Could you check a few things on this drawing? It's one solid part, dimensions in mm from its lowest x, y, z. A direction names the side the tool comes from. Give positions to 0.01 mm unless a question says otherwise; leave off trailing zeros. Order: outer loops, then holes, each group sorted by start corner. A loop starts at its lowest first (then second) coordinate and runs counter-clockwise, first axis right, second up. Notation, with made-up numbers: (77, -24) -> (131, -24) arc R10 cw to (131, -20) -> close; hole circle Ø7 at (-23.75, -9). An arc over 180 degrees is marked (long way). Write each question's results on one line, items separated by ' | '. Start each with the question number.
Q1. Imagine slicing it at C-C, the plane x = 65.5. Please give me the cut outline in (y, z).
Q2. Imagine slicing it at B-B, the plane y = 338.5. Please give me the cut outline in (x, z).
Q3. Thinking about a two-plate mould opening in Z: for the marked faces 1, 2, 3 and 4, which applies, pulls with the +Z half, pulls with the -Z half, needs draft (parallel to the pull), parting line crosses it, or undercut?
Q4. I need wall thicknesses on line 1 along Z through (x, y) = (708, 216.5); line 2 along X through (y, z) = (122, 313). Which ranges of each line are inside material? Lowest first, please. Write a range as [from, to].
Q5. I'm going to push a flat-ended pin straight in: pin 1 (3 mm diameter, centred on y = 198.5, z = 313, fed in from -X). Where does the tip first touch, or does it pass through?
Q6. For the marked faces 5 and 6, which set-ups out of +Z, -Z, +X, -X, +Y, -Y let a thin tool reach every point of the face, with its end or its side?
Q7. Imagine slicing it at A-A, the plane z = 424. Please give me the cut outline in (x, y).
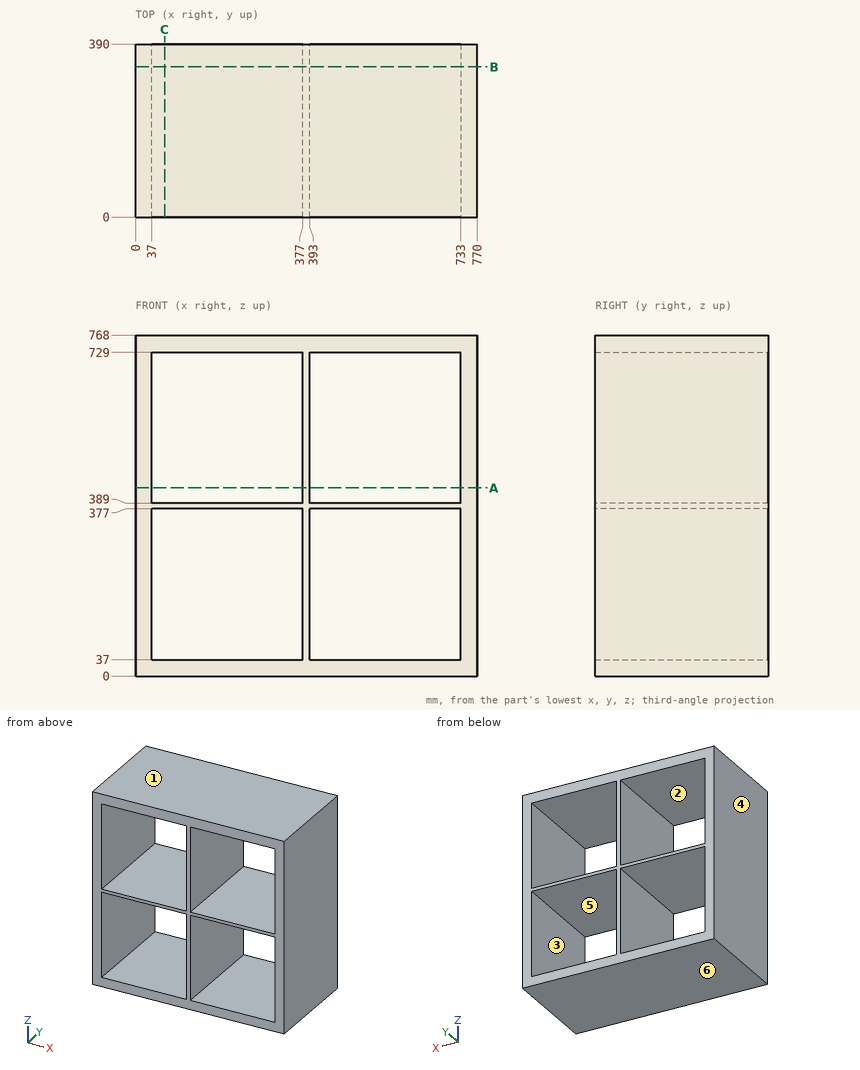
Geometry check:
1) outline: (0, 0) -> (390, 0) -> (390, 37) -> (0, 37) -> close; (0, 377) -> (390, 377) -> (390, 389) -> (0, 389) -> close; (0, 729) -> (390, 729) -> (390, 768) -> (0, 768) -> close
2) outline: (0, 0) -> (770, 0) -> (770, 768) -> (0, 768) -> close; hole (37, 37) -> (377, 37) -> (377, 377) -> (37, 377) -> close; hole (37, 389) -> (377, 389) -> (377, 729) -> (37, 729) -> close; hole (393, 37) -> (733, 37) -> (733, 377) -> (393, 377) -> close; hole (393, 389) -> (733, 389) -> (733, 729) -> (393, 729) -> close
3) face 1: pulls with the +Z half | face 2: undercut | face 3: undercut | face 4: needs draft
4) line 1: [0, 37], [377, 389], [729, 768] | line 2: [0, 37], [377, 393], [733, 770]
5) pin 1: x = 0
6) face 5: +Y, -Y | face 6: -Z, +X, -X, +Y, -Y
7) outline: (0, 0) -> (37, 0) -> (37, 390) -> (0, 390) -> close; (377, 0) -> (393, 0) -> (393, 390) -> (377, 390) -> close; (733, 0) -> (770, 0) -> (770, 390) -> (733, 390) -> close
